```python
from build123d import *

# Parameters (mm, degrees)
F1_DEPTH  = 120
F2_W      = 10
F2_H      = 10
F3_DEPTH  = 30
F5_DEPTH  = 30
F6_W      = 30
F6_H      = 100
F7_DEPTH  = 30
F9_DEPTH  = 60
F10_W     = 10
F10_H     = 10
F11_DEPTH = 30
F12_W     = 10
F12_H     = 10
F13_DEPTH = 30
F15_DEPTH = 30
F16_W     = 10
F16_H     = 23.5784614086
F17_DEPTH = 30


with BuildPart() as f1:
    # F0 (on Top) → F1 (new body)
    with BuildSketch(Plane.XY):
        Polygon((16.6459785789, 59.9448081851), (-33.3540214211, 59.9448081851), (-33.3540214211, 29.9448081851), (-33.3540214211, -50.0551918149), (-33.3540214211, -80.0551918149), (16.6459785789, -80.0551918149), (16.6459785789, -50.0551918149), (-3.3540214211, -50.0551918149), (-3.3540214211, 29.9448081851), (16.6459785789, 29.9448081851), align=None)
    extrude(amount=F1_DEPTH)

    # F2 (on face) → F3 (cut)
    with BuildSketch(Plane(origin=(0, 59.9448081851, 0), x_dir=(-1, 0, 0), z_dir=(0, 1, 0))):
        with Locations((-11.6459785789, 15)):
            Rectangle(F2_W, F2_H)
        with Locations((-1.6459785789, 25)):
            Rectangle(F2_W, F2_H)
        Polygon((-16.6459785789, 120), (-16.6459785789, 20), (-6.6459785789, 20), (-6.6459785789, 30), (3.3540214211, 30), (3.3540214211, 120), align=None)
    extrude(amount=-F3_DEPTH, mode=Mode.SUBTRACT)

    # F4 (on face) → F5 (cut)
    with BuildSketch(Plane.YZ.offset(-3.3540214211)):
        Polygon((-50.0551918149, 100), (29.9448081851, 20), (29.9448081851, 120), (-50.0551918149, 120), align=None)
    extrude(amount=-F5_DEPTH, mode=Mode.SUBTRACT)

    # F6 (on face) → F7 (cut)
    with BuildSketch(Plane.YZ.offset(-3.3540214211)):
        with Locations((44.9448081851, 70)):
            Rectangle(F6_W, F6_H)
    extrude(amount=-F7_DEPTH, mode=Mode.SUBTRACT)

    # F8 (on face) → F9 (cut)
    with BuildSketch(Plane(origin=(-33.3540214211, 0, 0), x_dir=(0, -1, 0), z_dir=(-1, 0, 0))):
        Polygon((50.0551918149, 80), (-29.9448081851, 0), (80.0551918149, 0), (80.0551918149, 80), align=None)
    extrude(amount=-F9_DEPTH, mode=Mode.SUBTRACT)

    # F10 (on face) → F11 (cut)
    with BuildSketch(Plane(origin=(-33.3540214211, 0, 0), x_dir=(0, -1, 0), z_dir=(-1, 0, 0))):
        with Locations((-24.9448081851, 25)):
            Rectangle(F10_W, F10_H)
        with Locations((45.0551918149, 95)):
            Rectangle(F10_W, F10_H)
        with Locations((35.0551918149, 85)):
            Rectangle(F10_W, F10_H)
        with Locations((25.0551918149, 75)):
            Rectangle(F10_W, F10_H)
        with Locations((15.0551918149, 65)):
            Rectangle(F10_W, F10_H)
        with Locations((5.0551918149, 55)):
            Rectangle(F10_W, F10_H)
        with Locations((-4.9448081851, 45)):
            Rectangle(F10_W, F10_H)
        with Locations((-14.9448081851, 35)):
            Rectangle(F10_W, F10_H)
    extrude(amount=-F11_DEPTH, mode=Mode.SUBTRACT)

    # F12 (on face) → F13 (cut)
    with BuildSketch(Plane.XZ.offset(80.0551918149)):
        with Locations((11.6459785789, 115)):
            Rectangle(F12_W, F12_H)
        with Locations((1.6459785789, 105)):
            Rectangle(F12_W, F12_H)
        Polygon((16.6459785789, 80), (16.6459785789, 100), (-3.5083531402, 88.195104599), (-3.5083531402, 80), align=None)
        with Locations((1.6459785789, 115)):
            Rectangle(F12_W, F12_H)
    extrude(amount=-F13_DEPTH, mode=Mode.SUBTRACT)

    # F14 (on face) → F15 (cut)
    with BuildSketch(Plane.XZ.offset(80.0551918149)):
        Polygon((-3.3540214211, 120), (-3.5083531402, 120), (-33.3540214211, 120), (-33.3540214211, 93.3674471554), (-3.3540214211, 93.3674471554), (-3.3540214211, 100), align=None)
    extrude(amount=-F15_DEPTH, mode=Mode.SUBTRACT)

    # F16 (on face) → F17 (cut)
    with BuildSketch(Plane.XZ.offset(80.0551918149)):
        with Locations((11.6459785789, 98.2107692957)):
            Rectangle(F16_W, F16_H)
    extrude(amount=-F17_DEPTH, mode=Mode.SUBTRACT)


solid = f1.part
```
Geometry check sheet. Reference: the model listing, model coordinates, mm. A direction names the side the tool comes from. Round coordinates to 2 decimals unless told otherwise and drop trailing zeros. Order: outer loops, then holes, each group sorted by start corner. A loop starts at its lowest first (then second) coordinate and runs counter-clockwise, first axis right, second up. Notation, with made-up numbers: M 88,11 L 117,11 A22 ccw 117,32 Z; hole C 39,-31.75 d2. An arc over 180 degrees is marked long. Write item = value, one per line.
Q1. Section check B-B (x = 3.5). Enter the section's corners in (y, z), plus the area to 3 significant figures.
Answer block:
outline = M -80.06,92.3 L -50.06,92.3 L -50.06,100 L -80.06,100 Z; M 29.94,0 L 59.94,0 L 59.94,20 L 29.94,20 Z
area = 831 mm^2
Q2. Section check A-A (x = -14). Enter the section's corners in (y, z).
Answer block:
outline = M -80.06,80 L -50.06,80 L 29.94,0 L 59.94,0 L 59.94,20 L 19.94,20 L 19.94,30 L 9.94,30 L 9.94,40 L -0.06,40 L -0.06,50 L -10.06,50 L -10.06,60 L -20.06,60 L -20.06,70 L -30.06,70 L -30.06,80 L -40.06,80 L -40.06,90 L -50.06,90 L -50.06,93.37 L -80.06,93.37 Z
Q3. Section check C-C (y = 46). Enter the section's corners in (x, z), plus the area to 3 significant figures.
Answer block:
outline = M -33.35,0 L 16.65,0 L 16.65,10 L 6.65,10 L 6.65,20 L -33.35,20 Z
area = 900 mm^2
Q4. Depth check by flat-ended pin: pin 1 Ø5 at (x, y) = (-22.5, -33) entering from +Z; pin 2 Ø3 at (x, z) = (-23, 33) entering from +Y; pin 3 Ø8 at (x, z) = (-20, 56.5) entering from +Y. Enter the tip coordinate at first touch or a pass-through.
Answer block:
pin_1 = 80
pin_2 = 9.94
pin_3 = -10.06
Q5. Set-up check for faces 1 (the flat face through (4, 29.945, 8)), 2 (the flat face through (-19, -30.055, 75)), 3 (the flat face through (-19, -65, 93.367)), 4 (the flat face through (-9, 45, 0)): record each of +Z, -Z, +X, -X, +Y, -Y from which the full face is reachable in a straight line by a thin tool's end or side.
Answer block:
face_1 = +Z, -Z, +X, -Y
face_2 = +Z, +X, -X, +Y
face_3 = +Z, -X, +Y, -Y
face_4 = -Z, +X, -X, +Y, -Y
Q6. Section check D-D (z = 24). Enter the section's corners in (x, y), plus the area to 3 significant figures.
Answer block:
outline = M -33.35,5.94 L -3.35,5.94 L -3.35,19.94 L -33.35,19.94 Z
area = 420 mm^2
Q7. Scan lines: line 1 (Z direction, x = -28.5, y = 36); line 2 (Y direction, x = 13.5, z = 4); line 3 (Z direction, x = -17, y = -71.5). Record each from-to range of solid material in increasing order.
Answer block:
line_1 = 0 to 20
line_2 = 29.94 to 59.94
line_3 = 80 to 93.37
